Build history of the part. All positions in model axes, mm. A direction names the side the tool comes from. Round coordinates to 2 decimals unless told otherwise and drop trailing zeros. Write each loop counter-clockwise with the first axis right and the second up, starting at its lowest first coordinate (ties: lowest second). Pieces come first, ordered by that corner, then holes. Notation, with made-up numbers: (-29.5, 67) - (6.5, 67) arc R12 cw to (6.5, 75) - close; hole circle Ø6 at (35.25, 74.25). An arc over 180 degrees is marked (long way). Write each question's results on one line, items separated by ' | '.
from build123d import *

# Parameters (mm, degrees)
EXTRUDE_5_DEPTH     = 0.8
EXTRUDE_6_DEPTH     = 0.28
EXTRUDE_8_DEPTH     = 0.84
SKETCH_1_9_R        = 0.5
CUT_EXTRUDE_1_DEPTH = 1.8
SKETCH_2_W          = 2.5
SKETCH_2_H          = 0.7
EXTRUDE_9_DEPTH     = 0.1


with BuildPart() as part:
    # Sketch 1 → Extrude 5 (new body)
    with BuildSketch(Plane.XY):
        with BuildLine():
            Line((-1.897366596, -4.3), (1.897366596, -4.3))
            ThreePointArc((1.897366596, -4.3), (3.323401872, -3.323401872), (4.3, -1.897366596))
            Line((4.3, -1.897366596), (4.3, 1.897366596))
            ThreePointArc((4.3, 1.897366596), (3.323401872, 3.323401872), (1.897366596, 4.3))
            Line((1.897366596, 4.3), (-1.897366596, 4.3))
            ThreePointArc((-1.897366596, 4.3), (-3.323401872, 3.323401872), (-4.3, 1.897366596))
            Line((-4.3, 1.897366596), (-4.3, -1.897366596))
            ThreePointArc((-4.3, -1.897366596), (-3.323401872, -3.323401872), (-1.897366596, -4.3))
        make_face()
    extrude(amount=EXTRUDE_5_DEPTH)

    # Sketch 1_6 → Extrude 6 (add)
    with BuildSketch(Plane.XY):
        Polygon((-0.919238816, 2.474873734), (-2.474873734, 0.919238816), (-3.889087297, 2.333452378), (-2.333452378, 3.889087297), align=None)
        Polygon((-1.626345597, 2.474873734), (-2.333452378, 3.181980515), (-3.181980515, 2.333452378), (-2.474873734, 1.626345597), align=None, mode=Mode.SUBTRACT)
        Polygon((2.474873734, 0.919238816), (3.889087297, 2.333452378), (2.333452378, 3.889087297), (0.919238816, 2.474873734), align=None)
        Polygon((2.474873734, 1.626345597), (3.181980515, 2.333452378), (2.333452378, 3.181980515), (1.626345597, 2.474873734), align=None, mode=Mode.SUBTRACT)
        Polygon((0.919238816, -2.474873734), (2.474873734, -0.919238816), (3.889087297, -2.333452378), (2.333452378, -3.889087297), align=None)
        Polygon((1.626345597, -2.474873734), (2.333452378, -3.181980515), (3.181980515, -2.333452378), (2.474873734, -1.626345597), align=None, mode=Mode.SUBTRACT)
        Polygon((-2.474873734, -0.919238816), (-0.919238816, -2.474873734), (-2.333452378, -3.889087297), (-3.889087297, -2.333452378), align=None)
        Polygon((-2.474873734, -1.626345597), (-3.181980515, -2.333452378), (-2.333452378, -3.181980515), (-1.626345597, -2.474873734), align=None, mode=Mode.SUBTRACT)
    extrude(amount=-EXTRUDE_6_DEPTH)

    # Sketch 1_8 → Extrude 8 (add)
    with BuildSketch(Plane.XY):
        Polygon((-1.626345597, 2.474873734), (-2.474873734, 1.626345597), (-3.181980515, 2.333452378), (-2.333452378, 3.181980515), align=None)
        Polygon((2.474873734, 1.626345597), (1.626345597, 2.474873734), (2.333452378, 3.181980515), (3.181980515, 2.333452378), align=None)
        Polygon((1.626345597, -2.474873734), (2.474873734, -1.626345597), (3.181980515, -2.333452378), (2.333452378, -3.181980515), align=None)
        Polygon((-2.474873734, -1.626345597), (-1.626345597, -2.474873734), (-2.333452378, -3.181980515), (-3.181980515, -2.333452378), align=None)
    extrude(amount=-EXTRUDE_8_DEPTH)

    # Sketch 1_9 → Cut-Extrude 1 (cut, through all)
    with BuildSketch(Plane.XY):
        with BuildLine():
            ThreePointArc((-2.25, -0.45), (-1.9, -0.8), (-1.55, -0.45))
            Line((-1.55, -0.45), (-1.55, 0.45))
            ThreePointArc((-1.55, 0.45), (-1.9, 0.8), (-2.25, 0.45))
            Line((-2.25, 0.45), (-2.25, -0.45))
        make_face()
        with BuildLine():
            Line((1.55, 0.45), (1.55, -0.45))
            ThreePointArc((1.55, -0.45), (1.9, -0.8), (2.25, -0.45))
            Line((2.25, -0.45), (2.25, 0.45))
            ThreePointArc((2.25, 0.45), (1.9, 0.8), (1.55, 0.45))
        make_face()
        Circle(SKETCH_1_9_R)
    extrude(amount=CUT_EXTRUDE_1_DEPTH, mode=Mode.SUBTRACT)

    # Sketch 2 → Extrude 9 (add)
    with BuildSketch(Plane.XY.offset(0.8)):
        with Locations((0, 3.5)):
            Rectangle(SKETCH_2_W, SKETCH_2_H)
        with Locations((0, 2)):
            Rectangle(SKETCH_2_W, SKETCH_2_H)
        with Locations((0, -2)):
            Rectangle(SKETCH_2_W, SKETCH_2_H)
        with Locations((0, -3.5)):
            Rectangle(SKETCH_2_W, SKETCH_2_H)
    extrude(amount=EXTRUDE_9_DEPTH)


solid = part.part
(1) Tool access for faces 1 (the flat face through (3, -3, -0.28)), 2 (the flat face through (-2.752, -2.764, -0.556)), 3 (the cylindrical face through (-3.341, -3.306, 0.394)): list every direction of +Z, -Z, +X, -X, +Y, -Y with a clear straight run to the whole face (end or side of a thin tool).
Worked answers:
face 1: -Z | face 2: -Z, -X, -Y | face 3: +Z, -Z, -X, -Y
(2) Drill centre lines: probe 1 along X at (y, z) = (0, 0.4); probe 2 along Y at (x, z) = (0, 0.5); probe 3 along Z at (x, y) = (-4, -1). Where is each one in solid material? Low to high. Write a range as [from, to].
Worked answers:
probe 1: x = [-4.3, -2.25], [-1.55, -0.5], [0.5, 1.55], [2.25, 4.3] | probe 2: y = [-4.3, -0.5], [0.5, 4.3] | probe 3: z = [0, 0.8]
(3) Two-plate mould, pull along X, no slides. Class faces 4 (the flat face through (2.752, 2.764, -0.556)), 5 (the flat face through (0, -1, 0)), 6 (the flat face through (2.4, -2.4, -0.84)): released by +X, released by -X, zero draft, split by the parting line, or undercut.
Worked answers:
face 4: released by +X | face 5: undercut | face 6: zero draft
(4) Slice it at A-A, the plane z = 0.1. Write the cut outline in (x, y), and give its area (3 significant figures).
Worked answers:
outline: (-4.3, -1.9) arc R4.7 ccw to (-1.9, -4.3) - (1.9, -4.3) arc R4.7 ccw to (4.3, -1.9) - (4.3, 1.9) arc R4.7 ccw to (1.9, 4.3) - (-1.9, 4.3) arc R4.7 ccw to (-4.3, 1.9) - close; hole (-2.25, -0.45) arc R0.35 ccw to (-1.55, -0.45) - (-1.55, 0.45) arc R0.35 ccw to (-2.25, 0.45) - close; hole circle Ø1 at (0, 0); hole (1.55, -0.45) arc R0.35 ccw to (2.25, -0.45) - (2.25, 0.45) arc R0.35 ccw to (1.55, 0.45) - close | area: 62.5 mm2
(5) Flat gauge pins, fed straight in: pin 1 Ø1 at (y, z) = (3, 0.5) entering from -X; pin 2 Ø3 at (x, y) = (-1.5, -1) entering from -Z. Where does each tip first touch, or does it go through?
Worked answers:
pin 1: stops at x = -3.98 | pin 2: stops at z = -0.84
(6) Slice it at C-C, the plane x = -2. Write the cut outline in (y, z), and give its area (3 significant figures).
Worked answers:
outline: (-4.25, 0) - (-3.56, 0) - (-3.56, -0.28) - (-2.85, -0.28) - (-2.85, -0.84) - (-2.1, -0.84) - (-2.1, -0.28) - (-1.39, -0.28) - (-1.39, 0) - (-0.79, 0) - (-0.79, 0.8) - (-4.25, 0.8) - close; (0.79, 0) - (1.39, 0) - (1.39, -0.28) - (2.1, -0.28) - (2.1, -0.84) - (2.85, -0.84) - (2.85, -0.28) - (3.56, -0.28) - (3.56, 0) - (4.25, 0) - (4.25, 0.8) - (0.79, 0.8) - close | area: 7.60 mm2
(7) Slice it at B-B, the plane y = 0. Write the cut outline in (x, z), and give its area (3 significant figures).
Worked answers:
outline: (-4.3, 0) - (-2.25, 0) - (-2.25, 0.8) - (-4.3, 0.8) - close; (-1.55, 0) - (-0.5, 0) - (-0.5, 0.8) - (-1.55, 0.8) - close; (0.5, 0) - (1.55, 0) - (1.55, 0.8) - (0.5, 0.8) - close; (2.25, 0) - (4.3, 0) - (4.3, 0.8) - (2.25, 0.8) - close | area: 4.96 mm2
(8) Slice it at D-D, the plane y = -2.75. Write the cut outline in (x, z).
Worked answers:
outline: (-3.81, 0) - (-3.47, 0) - (-3.47, -0.28) - (-2.77, -0.28) - (-2.77, -0.84) - (-1.9, -0.84) - (-1.9, -0.28) - (-1.19, -0.28) - (-1.19, 0) - (1.19, 0) - (1.19, -0.28) - (1.9, -0.28) - (1.9, -0.84) - (2.77, -0.84) - (2.77, -0.28) - (3.47, -0.28) - (3.47, 0) - (3.81, 0) - (3.81, 0.8) - (-3.81, 0.8) - close
